Check sheet for the modelled part. Datum: model origin and axes. Units: mm. A direction names the side the tool comes from. Give positions to 0.01 mm unless a question says otherwise; leave off trailing zeros. Loops run counter-clockwise (first coordinate to the right, second up) from the corner with the lowest first, then second, coordinate; pieces in that order, holes last. Notation, with made-up numbers: (-20.75, -33) - (22.25, -33) arc R7 ccw to (22.25, -20) - close; hole circle Ø6 at (30.5, -5.5). An arc over 180 degrees is marked (long way). Answer in a Markdown table with one row per item. Add a question column.
(1) Sectioned sample at D-D on x = 3.5. Enter the section's corners in (y, z), then the cut area to 3 significant figures.
(2) Draft check along X on faces 1 (the face through (1.784, 3.692, 5.916)), 2 (the face through (3, 3, 0)), 3 (the face through (-1, 10, 5)), 4 (the face through (-4, 6.8, 4.6)). Enter one of: released by +X, released by -X, zero draft, split by the parting line, or undercut.
(3) Sectioned sample at C-C on y = 0. Enter the section's corners in (x, z).
(4) Go/stop test with flat-tipped pins: P1, Ø12, axis at x = -8, y = -4, coming from the -Z side; P2, Ø5, axis at x = 4.5, z = 8, coming from the -Y side; P3, Ø3, axis at y = 8.11, z = 6, coming from the -X side; P4, Ø5.5, axis at y = 8.11, z = 6, coming from the +X side. Record where each tip stops, or that it passes through.
(5) Thickness scan on L1, parallel to X at y = 0, z = 1.75; L2, parallel to X at y = 1.5, z = 4.5; L3, parallel to Y at x = -2.7, z = 6. Record the ranges inside material, lowest first.
(6) Set-up check for faces 5 (the face through (-6.16, -9.73, 7.76)), 6 (the face through (-7.1, -9.2, 8.886)), 7 (the face through (1, 10, 5)): record each of +Z, -Z, +X, -X, +Y, -Y from which the full face is reachable in a straight line by a thin tool's end or side.
(7) Sectioned sample at B-B on z = 1.5. Enter the section's corners in (x, y), then the cut area to 3 significant figures.
(8) Sectioned sample at A-A on x = 8.6. Enter the section's corners in (y, z), then the cut area to 3 significant figures.
from build123d import *

# Parameters (mm, degrees)
BOSS_EXTRUDE1_DEPTH            = 12
SKETCH41_R                     = 1.7
CUT_EXTRUDE7_DEPTH             = 18
CBORE_FOR_M3_SHCS1_D           = 3.4
CBORE_FOR_M3_SHCS1_CBORE_D     = 6.5
CBORE_FOR_M3_SHCS1_CBORE_DEPTH = 3
F_3DSKETCH3_START              = 9
F_3DSKETCH3_OUTLINE_R          = 3.25
F_3DSKETCH3_OUTLINE_R_2        = 1.7
F_3DSKETCH3_DEPTH              = 3
CUT_EXTRUDE10_DEPTH            = 15
CUT_EXTRUDE10_DEPTH_BACK       = 15
SKETCH52_R                     = 1.7
SKETCH58_R                     = 3.25
CUT_EXTRUDE11_DEPTH            = 8
CUT_EXTRUDE12_DEPTH            = 4
CUT_EXTRUDE12_DEPTH_BACK       = 6
FILLET1_R                      = 2
SKETCH61_R                     = 3.25
CUT_EXTRUDE13_DEPTH            = 6
CUT_EXTRUDE14_DEPTH            = 1


# Read off the part's stored shape, not the designer's step: 3DSketch3
with BuildPart() as part:
    # Sketch1 → Boss-Extrude1 (new body)
    with BuildSketch(Plane(origin=(0, 0, 0), x_dir=(0, 1, 0), z_dir=(0, 0, 1))):
        with BuildLine():
            Line((-6.350852961, -13), (13.279056191, -13))
            Line((13.279056191, -13), (13.279056191, -1))
            Line((13.279056191, -1), (3.97617907, -1))
            ThreePointArc((3.97617907, -1), (3.68648689, -1.794384131), (3.24, -2.512449004))
            Line((3.24, -2.512449004), (-3.24, -2.512449004))
            ThreePointArc((-3.24, -2.512449004), (-3.879046275, -1.327780102), (-4.1, 0))
            ThreePointArc((-4.1, 0), (-0.503818326, 4.06892702), (3.97617907, 1))
            Line((3.97617907, 1), (13.279056191, 1))
            Line((13.279056191, 1), (13.279056191, 13))
            Line((13.279056191, 13), (-6.350852961, 13))
            Line((-6.350852961, 13), (-13.856406461, 0))
            Line((-13.856406461, 0), (-6.350852961, -13))
        make_face()
    extrude(amount=BOSS_EXTRUDE1_DEPTH)

    # Sketch41 → Cut-Extrude7 (cut)
    with BuildSketch(Plane(origin=(0, 0, 0), x_dir=(0, 1, 0), z_dir=(0, 0, 1))):
        with Locations(Location((0, 8.6, 0), (0, 0, 270))):
            Circle(SKETCH41_R)
        with Locations(Location((0, -8.6, 0), (0, 0, 270))):
            Circle(SKETCH41_R)
    extrude(amount=CUT_EXTRUDE7_DEPTH, mode=Mode.SUBTRACT)

    # CBORE for M3 SHCS1 (through all)
    with Locations(Plane(origin=(-8.6, 0, 12), x_dir=(1, 0, 0), z_dir=(0, 0, 1))):
        with Locations((0, 0)):
            CounterBoreHole(CBORE_FOR_M3_SHCS1_D / 2, CBORE_FOR_M3_SHCS1_CBORE_D / 2, CBORE_FOR_M3_SHCS1_CBORE_DEPTH)

    # 3DSketch3 outline → 3DSketch3 (cut)
    with BuildSketch(Plane.XY.offset(F_3DSKETCH3_START)):
        with Locations((8.6, 0)):
            Circle(F_3DSKETCH3_OUTLINE_R)
        with Locations((8.6, 0)):
            Circle(F_3DSKETCH3_OUTLINE_R_2, mode=Mode.SUBTRACT)
    extrude(amount=F_3DSKETCH3_DEPTH, mode=Mode.SUBTRACT)

    # Sketch52 → Cut-Extrude10 (cut, two sides: drawn at the far end of the back side and taken through both)
    with BuildSketch(Plane.YZ.offset(-1).offset(-CUT_EXTRUDE10_DEPTH_BACK)):
        with Locations((8.106406461, 6)):
            Circle(SKETCH52_R)
    extrude(amount=CUT_EXTRUDE10_DEPTH + CUT_EXTRUDE10_DEPTH_BACK, mode=Mode.SUBTRACT)

    # Sketch58 → Cut-Extrude11 (cut)
    with BuildSketch(Plane.YZ.offset(13)):
        with Locations(Location((8.106406461, 6, 0), (0, 0, 270))):
            Circle(SKETCH58_R)
    extrude(amount=-CUT_EXTRUDE11_DEPTH, mode=Mode.SUBTRACT)

    # Sketch60 → Cut-Extrude12 (cut, two sides: drawn at the far end of the back side and taken through both)
    with BuildSketch(Plane.YZ.offset(-8).offset(-CUT_EXTRUDE12_DEPTH_BACK)):
        Polygon((8.106406461, 2.709103466), (10.956406461, 4.354551733), (10.956406461, 7.645448267), (8.106406461, 9.290896534), (5.256406461, 7.645448267), (5.256406461, 4.354551733), align=None)
    extrude(amount=CUT_EXTRUDE12_DEPTH + CUT_EXTRUDE12_DEPTH_BACK, mode=Mode.SUBTRACT)

    # Fillet1
    # the kernel refuses this fillet: 2 mm, written as the material it takes off along each edge
    with BuildSketch(Plane(origin=(13, 13.279056191, -5), x_dir=(0, -1, 0), z_dir=(0, 0, 1)), Plane(origin=(-13, 13.279056191, -5), x_dir=(1, 0, 0), z_dir=(0, 0, 1))) as fillet1_piece_1:
        with BuildLine():
            CenterArc((FILLET1_R, -FILLET1_R), FILLET1_R, 90, 90)
            Line((0, -FILLET1_R), (0, 0))
            Line((0, 0), (FILLET1_R, 0))
        make_face()
    extrude(amount=22, mode=Mode.SUBTRACT)

    # Sketch61 → Cut-Extrude13 (cut)
    with BuildSketch(Plane(origin=(0, 0, 12), x_dir=(0, 1, 0), z_dir=(0, 0, 1))):
        with Locations(Location((0, 8.6, 0), (0, 0, 270))):
            Circle(SKETCH61_R)
        with Locations(Location((0, -8.6, 0), (0, 0, 270))):
            Circle(SKETCH61_R)
    extrude(amount=-CUT_EXTRUDE13_DEPTH, mode=Mode.SUBTRACT)

    # Sketch62 → Cut-Extrude14 (cut)
    with BuildSketch(Plane(origin=(-6, -10.392304845, 0), x_dir=(-0.8660254037844386, 0.5000000000000001, 0), z_dir=(-0.5000000000000001, -0.8660254037844386, 0))):
        Polygon((1.237336886, -6.103727624), (1.301138969, -6.103727624), (1.301138969, -8.526804547), (1.704985123, -8.526804547), (1.704985123, -8.885778906), (1.301138969, -8.885778906), (1.301138969, -9.693471213), (0.987036405, -9.693471213), (0.987036405, -8.885778906), (-0.673220005, -8.885778906), align=None)
        Polygon((0.987036405, -8.526804547), (0.987036405, -7.008174739), (-0.055531704, -8.526804547), align=None, mode=Mode.SUBTRACT)
    extrude(amount=-CUT_EXTRUDE14_DEPTH, mode=Mode.SUBTRACT)


solid = part.part
Reply:
| question | item | result |
|---|---|---|
| 1 | outline | (-11.84, 0) - (13.28, 0) - (13.28, 12) - (-11.84, 12) - close; hole circle Ø3.4 at (8.11, 6) |
| 1 | area | 292 mm^2 |
| 2 | face 1 | undercut |
| 2 | face 2 | zero draft |
| 2 | face 3 | undercut |
| 2 | face 4 | released by -X |
| 3 | outline | (-13, 0) - (-10.3, 0) - (-10.3, 6) - (-11.85, 6) - (-11.85, 12) - (-13, 12) - close; (-6.9, 0) - (-4.1, 0) - (-4.1, 12) - (-5.35, 12) - (-5.35, 6) - (-6.9, 6) - close; (2.51, 0) - (6.9, 0) - (6.9, 6) - (5.35, 6) - (5.35, 12) - (2.51, 12) - close; (10.3, 0) - (13, 0) - (13, 12) - (11.85, 12) - (11.85, 6) - (10.3, 6) - close |
| 4 | P1 | z = 0 |
| 4 | P2 | y = -12.7 |
| 4 | P3 | through |
| 4 | P4 | x = 5 |
| 5 | L1 | -13 to -10.3, -6.9 to -4.1, 2.51 to 6.9, 10.3 to 13 |
| 5 | L2 | -13 to -9.4, -7.8 to -3.82, 2.51 to 7.8, 9.4 to 13 |
| 5 | L3 | -12.3 to -3.09, 3.09 to 6.41, 9.81 to 13.28 |
| 6 | face 5 | none |
| 6 | face 6 | -Y |
| 6 | face 7 | +Z, -Z, +Y |
| 7 | outline | (-13, -6.35) - (0, -13.86) - (13, -6.35) - (13, 11.28) arc R2 ccw to (11, 13.28) - (1, 13.28) - (1, 3.98) arc R4.1 cw to (2.51, 3.24) - (2.51, -3.24) arc R4.1 cw (long way) to (-1, 3.98) - (-1, 13.28) - (-11, 13.28) arc R2 ccw to (-13, 11.28) - close; hole circle Ø3.4 at (-8.6, 0); hole circle Ø3.4 at (8.6, 0) |
| 7 | area | 524 mm^2 |
| 8 | outline | (-8.89, 0) - (-1.7, 0) - (-1.7, 6) - (-3.25, 6) - (-3.25, 12) - (-8.89, 12) - close; (1.7, 0) - (13.28, 0) - (13.28, 12) - (3.25, 12) - (3.25, 6) - (1.7, 6) - close; hole circle Ø6.5 at (8.11, 6) |
| 8 | area | 173 mm^2 |
